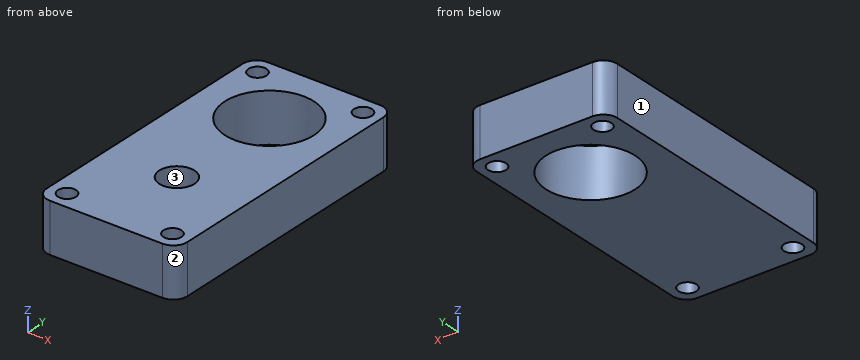
from build123d import *

# Parameters (mm, degrees)
SKETCH1_R           = 12.665
SKETCH1_R_2         = 2.554599
SKETCH1_R_3         = 5
BOSS_EXTRUDE1_DEPTH = 14
FILLET1_R           = 4
SKETCH11_R          = 7.5
BOSS_EXTRUDE3_DEPTH = 2


with BuildPart() as part:
    # Sketch1 → Boss-Extrude1 (new body)
    with BuildSketch(Plane.XY):
        Polygon((20, -10), (20, 20), (-20, 20), (-20, -10), (-20, -60), (20, -60), align=None)
        Circle(SKETCH1_R, mode=Mode.SUBTRACT)
        with Locations((-15, 15)):
            Circle(SKETCH1_R_2, mode=Mode.SUBTRACT)
        with Locations((15, 15)):
            Circle(SKETCH1_R_2, mode=Mode.SUBTRACT)
        with Locations((-15, -55)):
            Circle(SKETCH1_R_2, mode=Mode.SUBTRACT)
        with Locations((15, -55)):
            Circle(SKETCH1_R_2, mode=Mode.SUBTRACT)
        with Locations((0, -34)):
            Circle(SKETCH1_R_3, mode=Mode.SUBTRACT)
    extrude(amount=BOSS_EXTRUDE1_DEPTH)

    # Fillet1
    fillet1_edges = [part.edges().sort_by_distance(p)[0] for p in [
        (-20, 20, 7),
        (20, 20, 7),
        (20, -60, 7),
        (-20, -60, 7),
    ]]
    fillet(fillet1_edges, radius=FILLET1_R)

    # Sketch11 → Boss-Extrude3 (add)
    with BuildSketch(Plane(origin=(0, 0, 0), x_dir=(-1, 0, 0), z_dir=(0, 0, -1))):
        with Locations((0, -34)):
            Circle(SKETCH11_R)
    extrude(amount=-BOSS_EXTRUDE3_DEPTH)


solid = part.part
Model file for the job. Use its own axes, mm. Face numbers are marked on the shaded views. Round coordinates to 2 decimals unless told otherwise and drop trailing zeros. Order: outer loops, then holes, each group sorted by start corner. A loop starts at its lowest first (then second) coordinate and runs counter-clockwise, first axis right, second up.
(1) Band-saw the part on D-D (z = 4). List the corners of the cut face in (x, y) (3 decimals).
(2) Band-saw the part on C-C (x = 0). List the corners of the cut face in (y, z) (3 decimals).
(3) Pin check, flat tips, straight feed: pin 1 (5 mm diameter, centred on x = -1.5, y = -35.5, fed in from +Z); pin 2 (23 mm diameter, centred on x = 0, y = 0, fed in from -Z) (1 decimal). Stop position of each tip, or through.
(4) Band-saw the part on A-A (x = -15). List the corners of the cut face in (y, z).
(5) Band-saw the part on B-B (y = -55). List the corners of the cut face in (x, z).
(6) Drill centre lines: line 1 (Y direction, x = 15, z = 10); line 2 (Y direction, x = 0, z = 10.5) (3 decimals); line 3 (X direction, y = -53.5, z = 9.75). Where is each one in solid material? Low to high.
(7) Pull direction Y, two halves, no side cores. Call the marked faces 1, 2 and 3: released by +Y, released by -Y, zero draft, split by the parting line, or undercut.
Verdict:
1. outline: (-20, -56) arc R4 ccw to (-16, -60) - (16, -60) arc R4 ccw to (20, -56) - (20, 16) arc R4 ccw to (16, 20) - (-16, 20) arc R4 ccw to (-20, 16) - close; hole circle Ø5.109 at (-15, -55); hole circle Ø5.109 at (-15, 15); hole circle Ø25.33 at (0, 0); hole circle Ø10 at (0, -34); hole circle Ø5.109 at (15, -55); hole circle Ø5.109 at (15, 15)
2. outline: (-60, 0) - (-12.665, 0) - (-12.665, 14) - (-29, 14) - (-29, 2) - (-39, 2) - (-39, 14) - (-60, 14) - close; (12.665, 0) - (20, 0) - (20, 14) - (12.665, 14) - close
3. pin 1: stops at z = 2
3. pin 2: passes through
4. outline: (-60, 0) - (-57.55, 0) - (-57.55, 14) - (-60, 14) - close; (-52.45, 0) - (12.45, 0) - (12.45, 14) - (-52.45, 14) - close; (17.55, 0) - (20, 0) - (20, 14) - (17.55, 14) - close
5. outline: (-20, 0) - (-17.55, 0) - (-17.55, 14) - (-20, 14) - close; (-12.45, 0) - (12.45, 0) - (12.45, 14) - (-12.45, 14) - close; (17.55, 0) - (20, 0) - (20, 14) - (17.55, 14) - close
6. line 1: y = -60 to -57.55, -52.45 to 12.45, 17.55 to 20
6. line 2: y = -60 to -39, -29 to -12.665, 12.665 to 20
6. line 3: x = -20 to -17.07, -12.93 to 12.93, 17.07 to 20
7. face 1: zero draft
7. face 2: released by -Y
7. face 3: undercut
